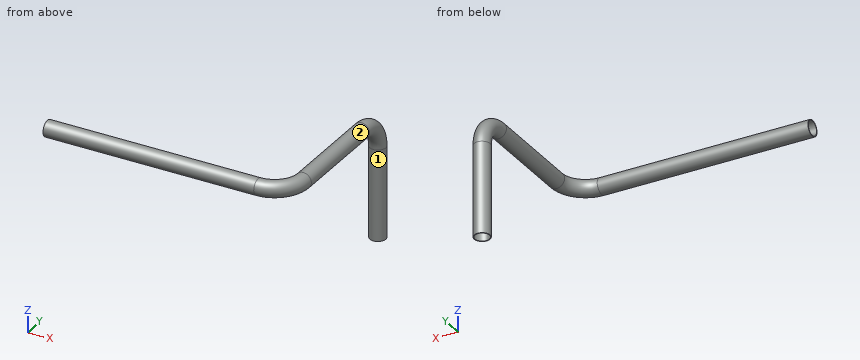
from build123d import *

# Parameters (mm, degrees)
SKIZZE1_R   = 10
SKIZZE1_R_2 = 9


with BuildPart() as part:
    # Austragung-Dünn1: sweep along a curve in space
    with BuildLine() as austragung_d_nn1_path:
        Line((0, 0, 0), (264, 0, 0))
        ThreePointArc((264, 0, 0), (289.455844123, 10.544155877, 0), (300, 36, 0))
        Line((300, 36, 0), (300, 164, 0))
        ThreePointArc((300, 164, 0), (300, 189.455844123, -10.544155877), (300, 200, -36))
        Line((300, 200, -36), (300, 200, -150))
    # Skizze1 → Austragung-Dünn1 (sweep)
    with BuildSketch(Plane(origin=(0, 0, 0), x_dir=(0, 0, -1), z_dir=(1, 0, 0))):
        Circle(SKIZZE1_R)
        Circle(SKIZZE1_R_2, mode=Mode.SUBTRACT)
    sweep(path=austragung_d_nn1_path.line)


solid = part.part
Geometry: final body of the model. Coordinates: model frame, mm. Face numbers are marked on the shaded views. Coordinates: 2 decimals unless noted, no trailing zeros. Loops run counter-clockwise (first coordinate to the right, second up) from the corner with the lowest first, then second, coordinate; pieces in that order, holes last. Notation, with made-up numbers: M 31.25,61.5 L 69.25,61.5 A35 ccw 69.25,96.5 Z; hole C 10,-23 d5. An arc over 180 degrees is marked long. One line per item, written item: value. Start each with the question number.
1) Material intervals for L1, parallel to Z at x = 300, y = 110; L2, parallel to X at y = 200, z = -58, sorted ascending. Write a range as from..to.
2) Draft query along Y for the marked faces 1 and 2. Return one class per face: released by +Y, released by -Y, zero draft, split by the parting line, or undercut.
3) Cut plane B-B (y = 49.5). Return loops of the section in (x, z), then the cut area to 3 significant figures.
4) Cut plane A-A (x = 172.5). Return loops of the section in (y, z).
5) Pin query (flat end, axial travel): P1, Ø11, axis at x = 300, z = 0, coming from the +Y side; P2, Ø20.5, axis at y = 0, z = 0, coming from the +X side. Return the tip coordinate at first contact, or that it passes through.
Evaluation:
1. L1: -10..-9, 9..10
1. L2: 290..291, 309..310
2. face 1: split by the parting line
2. face 2: undercut
3. outline: C 300,0 d20; hole C 300,0 d18
3. area: 59.7 mm^2
4. outline: C 0,0 d20; hole C 0,0 d18
5. P1: y = 198.43
5. P2: x = 302.12
